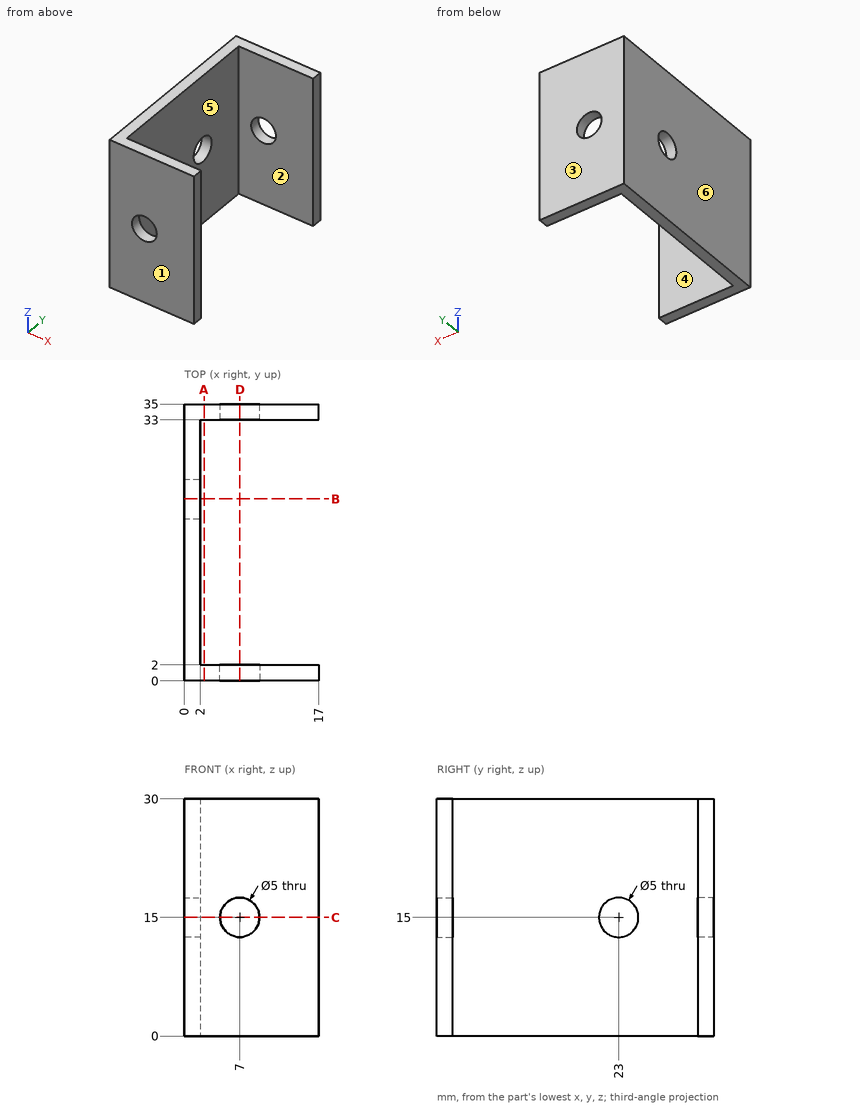
Verification items for this drawing (mm, ordinates from the low corner). A direction names the side the tool comes from. Coordinates: 2 decimals unless noted, no trailing zeros. Order: outer loops, then holes, each group sorted by start corner. A loop starts at its lowest first (then second) coordinate and runs counter-clockwise, first axis right, second up. Notation, with made-up numbers: M 41,74 L 73,74 A20 ccw 73,89 Z; hole C -16,-9 d2. An arc over 180 degrees is marked long. Answer as a JSON object with one key per item and string values.
Q1. Depth check by flat-ended pin: pin 1 Ø6 at (y, z) = (16.5, 5) entering from +X. Enter the tip coordinate at first touch or a pass-through.
Results are:
{"pin 1": "stops at x = 2"}
Q2. Tool access check on the marked faces 1 and 2. Record the directions out of +Z, -Z, +X, -X, +Y, -Y that give a thin tool (end or side, any length) a straight path to the whole face; none if there is none.
Results are:
{"face 1": "+Z, -Z, +X, -X, -Y", "face 2": "+Z, -Z, +X"}
Q3. Cross-section at C-C on z = 15. Record the cut outline in (x, y).
Results are:
{"outline": "M 0,0 L 4.5,0 L 4.5,2 L 2,2 L 2,20.5 L 0,20.5 Z; M 0,25.5 L 2,25.5 L 2,33 L 4.5,33 L 4.5,35 L 0,35 Z; M 9.5,0 L 17,0 L 17,2 L 9.5,2 Z; M 9.5,33 L 17,33 L 17,35 L 9.5,35 Z"}
Q4. Release check for a two-part mould opening along Y. For the marked faces 3, 4, 5 and 6 record: released by +Y, released by -Y, zero draft, split by the parting line, or undercut.
Results are:
{"face 3": "released by +Y", "face 4": "undercut", "face 5": "undercut", "face 6": "zero draft"}
Q5. Cross-section at B-B on y = 23. Record the cut outline in (x, z).
Results are:
{"outline": "M 0,0 L 2,0 L 2,12.5 L 0,12.5 Z; M 0,17.5 L 2,17.5 L 2,30 L 0,30 Z"}
Q6. Cross-section at D-D on x = 7. Record the cut outline in (y, z), and give its area (3 significant figures).
Results are:
{"outline": "M 0,0 L 2,0 L 2,12.5 L 0,12.5 Z; M 0,17.5 L 2,17.5 L 2,30 L 0,30 Z; M 33,0 L 35,0 L 35,12.5 L 33,12.5 Z; M 33,17.5 L 35,17.5 L 35,30 L 33,30 Z", "area": "100 mm²"}
Q7. Scan lines: line 1 (Y direction, x = 8.25, z = 20); line 2 (Z direction, x = 7, y = 1.5); line 3 (X direction, y = 14, z = 16.5). Record each from-to range of solid material in increasing order.
Results are:
{"line 1": "y = 0 to 2, 33 to 35", "line 2": "z = 0 to 12.5, 17.5 to 30", "line 3": "x = 0 to 2"}
Q8. Cross-section at A-A on x = 2.5. Record the cut outline in (y, z), and give its area (3 significant figures).
Results are:
{"outline": "M 0,0 L 2,0 L 2,30 L 0,30 Z; M 33,0 L 35,0 L 35,30 L 33,30 Z", "area": "120 mm²"}
